Autodesk Fusion 360 part; units mm, degrees
sketch "Sketch1" plane through (0, 0, 0) normal (0, 0, 1) x (1, 0, 0)
  circle A0 centre (0, 0) radius 4
  circle A1 centre (0, 0) radius 5
  dimension "d1" = 8
  dimension "d2" = 1
extrude "Extrude1" add sketch "Sketch1" along normal blind 3
extrude "Extrude2" add sketch "Sketch1" along normal blind 6 contours A0
sketch "Sketch2" plane through (0, 0, 6) normal (0, 0, 1) x (-1, 0, 0)
  circle A0 centre (0, 0) radius 4
  circle A1 centre (-2, 2) radius 0.5
  circle A2 centre (0, 2) radius 0.5
  circle A3 centre (2, 2) radius 0.5
  circle A4 centre (-2, 0) radius 0.5
  circle A5 centre (0, 0) radius 0.5
  circle A6 centre (2, 0) radius 0.5
  circle A7 centre (-2, -2) radius 0.5
  circle A8 centre (0, -2) radius 0.5
  circle A9 centre (2, -2) radius 0.5
  point P0 (-2, 2)
  dimension "d7" = 1
  dimension "d8" = 1
  dimension "d9" = 1
  dimension "d10" = 1
  dimension "d11" = 1
  dimension "d12" = 1
  dimension "d13" = 1
  dimension "d14" = 1
  dimension "d15" = 1
hole "Hole1" at (2, -2, 6) at (0, -2, 6) at (-2, -2, 6) at (2, 0, 6) at (0, 0, 6) at (-2, 0, 6) at (2, 2, 6) at (0, 2, 6) at (-2, 2, 6) direction (0, 0, -1) diameter 1 depth 6 tip angle 180
Design review of the part built by this model. Coordinates are the model's own, in mm. A direction names the side the tool comes from. Round coordinates to 2 decimals unless told otherwise and drop trailing zeros. Order: outer loops, then holes, each group sorted by start corner. A loop starts at its lowest first (then second) coordinate and runs counter-clockwise, first axis right, second up.
1) Consider section C-C (x = 1.75). State the section outline as (y, z) points.
The answers:
outline: (-4.68, 0) - (-2.43, 0) - (-2.43, 6) - (-3.6, 6) - (-3.6, 3) - (-4.68, 3) - close; (-1.57, 0) - (-0.43, 0) - (-0.43, 6) - (-1.57, 6) - close; (0.43, 0) - (1.57, 0) - (1.57, 6) - (0.43, 6) - close; (2.43, 0) - (4.68, 0) - (4.68, 3) - (3.6, 3) - (3.6, 6) - (2.43, 6) - close
2) Consider section A-A (y = 0). State the section outline as (x, z) points, plus the area to 3 significant figures.
The answers:
outline: (-5, 0) - (-2.5, 0) - (-2.5, 6) - (-4, 6) - (-4, 3) - (-5, 3) - close; (-1.5, 0) - (-0.5, 0) - (-0.5, 6) - (-1.5, 6) - close; (0.5, 0) - (1.5, 0) - (1.5, 6) - (0.5, 6) - close; (2.5, 0) - (5, 0) - (5, 3) - (4, 3) - (4, 6) - (2.5, 6) - close
area: 36.0 mm2
3) Machinability: for faces 4 (the cylindrical face through (1.504, 0.065, 2.958)), 5 (the cylindrical face through (-0.867, 3.905, 4.479)), which of the approach directions +Z, -Z, +X, -X, +Y, -Y give a long, thin tool a straight path to every point of the face, cutting with its end or side? Answer none if there is none.
The answers:
face 4: +Z, -Z
face 5: +Z
4) Consider section B-B (z = 4.9). Count the separate pieces of the cut face and the enclosed holes in it, plus the area to 3 significant figures.
The answers:
separate pieces: 1
enclosed holes: 9
area: 43.2 mm2
5) Draft analysis for pull direction X (two halves, no side actions). For faces 1 (the cylindrical face through (-1.08, 4.88, 1.48)), 2 (the cylindrical face through (0.488, 0.108, 2.958)), 3 (the flat face through (0, -1, 6)), state which applies: released by +X, released by -X, zero draft, split by the parting line, or undercut.
The answers:
face 1: split by the parting line
face 2: undercut
face 3: zero draft
6) Clearance check with flat-ended pins moving along their axes: pin 1 Ø1.5 at (x, z) = (-1.5, 1.5) entering from -Y; pin 2 Ø1.5 at (y, z) = (2.5, 1.5) entering from +X. State where each tip first meets the part, or that it passes through.
The answers:
pin 1: stops at y = -4.94
pin 2: stops at x = 4.68
7) For L1, parallel to Y at x = -0.25, z = 1.15; L2, parallel to Y at x = 0, z = 2.9; L3, parallel to X at y = 2, z = 1.9, list the stretches that pass through material, from the lowest coordinate up.
The answers:
L1: y = -4.99 to -2.43, -1.57 to -0.43, 0.43 to 1.57, 2.43 to 4.99
L2: y = -5 to -2.5, -1.5 to -0.5, 0.5 to 1.5, 2.5 to 5
L3: x = -4.58 to -2.5, -1.5 to -0.5, 0.5 to 1.5, 2.5 to 4.58
